from build123d import *

# Parameters (mm, degrees)
F2_W     = 30
F2_H     = 3
F4_R     = 5
F5_DEPTH = 61.201
F6_R     = 2
F7_DEPTH = 260.001
F8_R     = 3
F9_DEPTH = 61.201


with BuildPart() as f3:
    # F3: sweep along a path in F0
    with BuildLine(Plane.XZ) as f3_path:
        Line((-258.5, 29.1), (-5, 29.1))
        ThreePointArc((-5, 29.1), (-1.4644660941, 27.6355339059), (0, 24.1))
        Line((0, 24.1), (0, -24.1))
        ThreePointArc((0, -24.1), (-1.4644660941, -27.6355339059), (-5, -29.1))
        Line((-5, -29.1), (-258.5, -29.1))
    # F2 (on plane+point) → F3 (sweep)
    with BuildSketch(Plane.YZ.offset(-258.5)):
        with Locations((0, 29.1)):
            Rectangle(F2_W, F2_H)
    sweep(path=f3_path.line)

    # F4 (on face) → F5 (cut, through all)
    with BuildSketch(Plane(origin=(0, 0, -30.6), x_dir=(1, 0, 0), z_dir=(0, 0, -1))):
        with Locations((-89, 0)):
            Circle(F4_R)
    extrude(amount=-F5_DEPTH, mode=Mode.SUBTRACT)

    # F6 (on face) → F7 (cut, through all)
    with BuildSketch(Plane.YZ.offset(1.5)):
        with Locations((0, 10)):
            Circle(F6_R)
        with Locations((0, -10)):
            Circle(F6_R)
    extrude(amount=-F7_DEPTH, mode=Mode.SUBTRACT)

    # F8 (on face) → F9 (cut, through all)
    with BuildSketch(Plane(origin=(0, 0, -30.6), x_dir=(1, 0, 0), z_dir=(0, 0, -1))):
        with Locations((-243.5, 0)):
            Circle(F8_R)
    extrude(amount=-F9_DEPTH, mode=Mode.SUBTRACT)


solid = f3.part
Here's how the part is built. I have some questions about the finished solid (model axes, mm). A direction names the side the tool comes from. Give positions to 0.01 mm unless a question says otherwise; leave off trailing zeros. Write each loop counter-clockwise with the first axis right and the second up, starting at its lowest first coordinate (ties: lowest second). Pieces come first, ordered by that corner, then holes. Notation, with made-up numbers: (-9, 13.5) -> (41, 13.5) arc R28 cw to (41, 43.5) -> close; hole circle Ø4 at (-3, 85.25). An arc over 180 degrees is marked (long way). Use one line per item in the form item = value. Start each with the question number.
1. If I drill on L1, parallel to Z at x = -234, y = 10; L2, parallel to Y at x = -243.5, z = 29.6; L3, parallel to X at y = 0, z = 29.05, over which ranges is the centre line in solid material (lowest first)?
2. On a 3-axis mill with a long thin cutter (end or side, diameter ignored), from which of +Z, -Z, +X, -X, +Y, -Y can I reach the whole of each face in a straight line? I mean faces 1 (the face through (-134, 0, -27.6)), 2 (the face through (1.5, 0, 0)). Say none if no direction works.
3. Imagine slicing it at B-B on x = -190. List the corners of the cut face in (y, z) for me.
4. Imagine slicing it at C-C on y = 12.75. List the corners of the cut face in (x, z) for me, plus the area to 3 significant figures.
5. Thinking about a two-plate mould opening in Y: for faces 3 (the face through (-246.5, -0.1, 29.1)), 4 (the face through (-0.354, -0.21, -28.645)), 5 (the face through (-84.381, 1.915, 29.079)), 6 (the face through (-128, -15, 30)), which applies, +Y half, -Y half, draft (parallel to the pull), parting line (faces both ways), or undercut?
6. Will these pins go through, and if not, where does the flat tip stop? pin 1 Ø5 at (y, z) = (0, 10) entering from -X; pin 2 Ø8 at (y, z) = (-9, -21.5) entering from -X.
7. Imagine slicing it at D-D on x = -243.5. List the corners of the cut face in (y, z) for me, plus the area to 3 significant figures.
8. Imagine slicing it at A-A on x = -89. List the corners of the cut face in (y, z) for me.
Entries:
q1.L1 = -30.6 to -27.6, 27.6 to 30.6
q1.L2 = -15 to -3, 3 to 15
q1.L3 = -258.5 to -246.5, -240.5 to -94, -84 to -0.79
q2.face_1 = -X, +Y, -Y
q2.face_2 = +Z, -Z, +X, +Y, -Y
q3.outline = (-15, -30.6) -> (15, -30.6) -> (15, -27.6) -> (-15, -27.6) -> close; (-15, 27.6) -> (15, 27.6) -> (15, 30.6) -> (-15, 30.6) -> close
q4.outline = (-258.5, -30.6) -> (-5, -30.6) arc R6.5 ccw to (1.5, -24.1) -> (1.5, 24.1) arc R6.5 ccw to (-5, 30.6) -> (-258.5, 30.6) -> (-258.5, 27.6) -> (-5, 27.6) arc R3.5 cw to (-1.5, 24.1) -> (-1.5, -24.1) arc R3.5 cw to (-5, -27.6) -> (-258.5, -27.6) -> close
q4.area = 1,710 mm²
q5.face_3 = undercut
q5.face_4 = draft
q5.face_5 = undercut
q5.face_6 = -Y half
q6.pin_1 = -1.5
q6.pin_2 = -1.79
q7.outline = (-15, -30.6) -> (-3, -30.6) -> (-3, -27.6) -> (-15, -27.6) -> close; (-15, 27.6) -> (-3, 27.6) -> (-3, 30.6) -> (-15, 30.6) -> close; (3, -30.6) -> (15, -30.6) -> (15, -27.6) -> (3, -27.6) -> close; (3, 27.6) -> (15, 27.6) -> (15, 30.6) -> (3, 30.6) -> close
q7.area = 144 mm²
q8.outline = (-15, -30.6) -> (-5, -30.6) -> (-5, -27.6) -> (-15, -27.6) -> close; (-15, 27.6) -> (-5, 27.6) -> (-5, 30.6) -> (-15, 30.6) -> close; (5, -30.6) -> (15, -30.6) -> (15, -27.6) -> (5, -27.6) -> close; (5, 27.6) -> (15, 27.6) -> (15, 30.6) -> (5, 30.6) -> close
